CAD build for the part. Positions are in the model's coordinates, mm. A direction names the side the tool comes from. Coordinates: 2 decimals unless noted, no trailing zeros. Write each loop counter-clockwise with the first axis right and the second up, starting at its lowest first coordinate (ties: lowest second). Pieces come first, ordered by that corner, then holes. Notation, with made-up numbers: (-31, -40) - (-26, -40) arc R18 cw to (-26, -7) - close; hole circle Ø3 at (14, -11.5). An arc over 180 degrees is marked (long way). Answer in a Markdown table with one row per item. Add a question column.
Q1. 3-axis set-ups, long thin cutter, end or side, ignore diameter. For faces 4 (the cylindrical face through (-44.229, -0.057, 96.297)), 5 (the flat face through (5, 13.125, 20)), 6 (the flat face through (34, 34, 61)): which of +Z, -Z, +X, -X, +Y, -Y reach the whole face in a straight line?
Q2. Band-saw the part on A-A (z = 54). List the corners of the cut face in (x, y), and give its area (3 significant figures).
Q3. Band-saw the part on C-C (z = 16). List the corners of the cut face in (x, y).
Q4. Band-saw the part on B-B (y = 6.5). List the corners of the cut face in (x, z).
Q5. Two-plate mould, pull along X, no slides. Class faces 1 (the cylindrical face through (29.219, 0.307, 23.004)), 2 (the flat face through (34, 34, 41)), 3 (the flat face through (130.71, 85.75, 50.29)): +X half, -X half, draft (parallel to the pull), parting line (faces both ways), or undercut.
Q6. Drill centre lines: line 1 along X through (y, z) = (6.5, 27); line 2 along X through (y, z) = (12, 87); line 3 along Y through (x, z) = (-10.5, 92). Where is each one in solid material? Low to high. Write a range as from..to.
Q7. Pin check, flat tips, straight feed: pin 1 (2 mm diameter, centred on x = 164.5, z = 25.5, fed in from +Y); pin 2 (1 mm diameter, centred on y = 75, z = 11.5, fed in from -X); pin 3 (8 mm diameter, centred on x = 118.5, z = 48, fed in from +Y); pin 4 (16 mm diameter, centred on x = -30.24, z = 20, fed in from -Y). Stop position of each tip, or through.
Q8. Band-saw the part on D-D (x = 62.5). List the corners of the cut face in (y, z), and give its area (3 significant figures).
```python
from build123d import *

# Parameters (mm, degrees)
F1_DEPTH  = 102
F2_R      = 50.99999
F3_R      = 27
F3_R_2    = 18.5
F4_DEPTH  = 30
F7_DEPTH  = 10
F8_R      = 18.5
F9_DEPTH  = 26
F10_R     = 20
F11_R     = 10
F12_DEPTH = 26


# Not quite as in the source:
# - a fillet or chamfer is up to 0.001 mm smaller than in the source, because OpenCascade refuses the exact size


with BuildPart() as f1:
    # F0 (on Top) → F1 (new body)
    with BuildSketch(Plane.XY):
        Polygon((-50.2432771027, 13.1253414819), (-50.2432771027, -12.8746585181), (73.7678298962, -12.8746585181), (189.2678298962, 187.1772097561), (166.7511693978, 200.1772097561), (58.7567228973, 13.1253414819), align=None)
    extrude(amount=F1_DEPTH)

    # F2 (radius 51 in the source; OpenCascade refuses exactly that, so slightly less here)
    f2_edges = [f1.edges().sort_by_distance(p)[0] for p in [
        (178.0095, 193.67721, 0),
        (178.0095, 193.67721, 102),
    ]]
    fillet(f2_edges, radius=F2_R)

    # F3 (on face) → F4 (join)
    with BuildSketch(Plane(origin=(38.3841025946, -22.1610719656, 0), x_dir=(-0.5, -0.8660254038, 0), z_dir=(-0.8660254038, 0.5, 0))):
        with Locations((-205.7341336064, 51)):
            Circle(F3_R)
        with Locations((-205.7341336064, 51)):
            Circle(F3_R_2, mode=Mode.SUBTRACT)
    extrude(amount=F4_DEPTH)

    # F6 (on offset) → F7 (join, symmetric)
    with BuildSketch(Plane.XY.offset(51)):
        Polygon((96.7567228973, 78.9432721695), (-50.2432771027, 13.1253414819), (58.7567228973, 13.1253414819), align=None)
    extrude(amount=F7_DEPTH, both=True)

    # F8 (on face) → F9 (cut)
    with BuildSketch(Plane(origin=(38.3841025946, -22.1610719656, 0), x_dir=(-0.5, -0.8660254038, 0), z_dir=(-0.8660254038, 0.5, 0))):
        with Locations((-205.7341336064, 51)):
            Circle(F8_R)
    extrude(amount=-F9_DEPTH, mode=Mode.SUBTRACT)

    # F10
    f10_edges = [f1.edges().sort_by_distance(p)[0] for p in [
        (-50.243277, 0.125341, 0),
        (-50.243277, 0.125341, 102),
    ]]
    fillet(f10_edges, radius=F10_R)

    # F11 (on face) → F12 (cut)
    with BuildSketch(Plane(origin=(0, 13.1253414819, 0), x_dir=(-1, 0, 0), z_dir=(0, 1, 0))):
        with Locations((30.2432771027, 20)):
            Circle(F11_R)
        with Locations((30.2432771027, 82)):
            Circle(F11_R)
        with Locations((-38.7567228973, 20)):
            Circle(F11_R)
        with Locations((-38.7567228973, 82)):
            Circle(F11_R)
    extrude(amount=-F12_DEPTH, mode=Mode.SUBTRACT)


solid = f1.part
```
Checked values:
| question | item | result |
|---|---|---|
| 1 | face 4 | +Z, -X, +Y, -Y |
| 1 | face 5 | -Z, -X, +Y |
| 1 | face 6 | +Z, -X, +Y |
| 2 | outline | (-50.24, -12.87) - (73.77, -12.87) - (154.64, 127.2) - (106.14, 155.2) - (101.85, 147.77) - (127.83, 132.77) - (96.76, 78.94) - (-50.24, 13.13) - close; (124.4, 186.82) - (172.9, 158.82) - (189.22, 187.1) - (166.71, 200.1) - (154.67, 179.25) - (128.69, 194.25) - close |
| 2 | area | 12,000 mm² |
| 3 | outline | (-49.84, -12.87) - (-39.41, -12.87) - (-39.41, 13.13) - (-49.84, 13.13) - close; (-21.08, -12.87) - (29.59, -12.87) - (29.59, 13.13) - (-21.08, 13.13) - close; (47.92, -12.87) - (73.77, -12.87) - (182.32, 175.13) - (159.8, 188.13) - (58.76, 13.13) - (47.92, 13.13) - close |
| 4 | outline | (-50.24, 20) arc R20 ccw to (-30.24, 0) - (84.95, 0) - (84.95, 102) - (-30.24, 102) arc R20 ccw to (-50.24, 82) - close; hole circle Ø20 at (-30.24, 20); hole circle Ø20 at (-30.24, 82); hole circle Ø20 at (38.76, 20); hole circle Ø20 at (38.76, 82) |
| 5 | face 1 | undercut |
| 5 | face 2 | draft |
| 5 | face 3 | +X half |
| 6 | line 1 | x = -50.24..-37.38, -23.1..31.62, 45.9..84.95 |
| 6 | line 2 | x = -49.61..-38.9, -21.58..30.1, 47.42..88.13 |
| 6 | line 3 | y = -12.87..13.13 |
| 7 | pin 1 | stops at y = 194.46 |
| 7 | pin 2 | stops at x = 94.19 |
| 7 | pin 3 | stops at y = 150.58 |
| 7 | pin 4 | passes through |
| 8 | outline | (-12.87, 0) - (19.61, 0) - (19.61, 41) - (63.61, 41) - (63.61, 61) - (19.61, 61) - (19.61, 102) - (-12.87, 102) - close |
| 8 | area | 4,190 mm² |
